Source: CAD feature listing. Evaluate the final solid. Frame: model axes, mm. A direction names the side the tool comes from. Round coordinates to 2 decimals unless told otherwise and drop trailing zeros. Loops run counter-clockwise (first coordinate to the right, second up) from the corner with the lowest first, then second, coordinate; pieces in that order, holes last. Notation, with made-up numbers: M 60.5,-33 L 101.5,-33 A22 cw 101.5,-17 Z; hole C -23,9 d10. An arc over 180 degrees is marked long. Answer as CSV lines item,"result". Start each with the question number.
```python
from build123d import *

# Parameters (mm, degrees)
SKETCH1_W           = 406.4
SKETCH1_H           = 431.8
SKETCH1_W_2         = 355.6
SKETCH1_H_2         = 381
BOSS_EXTRUDE1_DEPTH = 304.8
SKETCH2_W           = 254
SKETCH2_H           = 381
CUT_EXTRUDE1_DEPTH  = 552.975370827
BOSS_EXTRUDE2_DEPTH = 101.6
SKETCH4_W           = 25.4
SKETCH4_H           = 76.2
BOSS_EXTRUDE3_DEPTH = 533.4
BOSS_EXTRUDE4_DEPTH = 25.4
BOSS_EXTRUDE5_DEPTH = 25.4
SKETCH7_W           = 152.4
SKETCH7_H           = 25.4
BOSS_EXTRUDE6_DEPTH = 292.1
SKETCH8_R           = 4.7625
SKETCH8_R_2         = 7
CUT_EXTRUDE2_DEPTH  = 25.4
SKETCH9_R           = 12.7
CUT_EXTRUDE3_DEPTH  = 12.7
BOSS_EXTRUDE7_DEPTH = 25.4
SKETCH11_W          = 304.8
SKETCH11_H          = 25.4
BOSS_EXTRUDE8_DEPTH = 63.5
SKETCH12_W          = 304.8
SKETCH12_H          = 25.4
BOSS_EXTRUDE9_DEPTH = 63.5
SKETCH14_R          = 9.525
CUT_EXTRUDE4_DEPTH  = 830.495714275
SKETCH16_W          = 300
SKETCH16_H          = 160
CUT_EXTRUDE5_DEPTH  = 30


with BuildPart() as part:
    # Sketch1 → Boss-Extrude1 (new body)
    with BuildSketch(Plane.XY):
        Rectangle(SKETCH1_W, SKETCH1_H)
        Rectangle(SKETCH1_W_2, SKETCH1_H_2, mode=Mode.SUBTRACT)
    extrude(amount=BOSS_EXTRUDE1_DEPTH)

    # Sketch2 → Cut-Extrude1 (cut, through all)
    with BuildSketch(Plane(origin=(203.2, 0, 0), x_dir=(0, 0, -1), z_dir=(1, 0, 0))):
        with Locations((-177.8, 0)):
            Rectangle(SKETCH2_W, SKETCH2_H)
    extrude(amount=-CUT_EXTRUDE1_DEPTH, mode=Mode.SUBTRACT)

    # Sketch3 → Boss-Extrude2 (add)
    with BuildSketch(Plane(origin=(0, 215.9, 0), x_dir=(1, 0, 0), z_dir=(0, 1, 0))):
        Polygon((-57.785, 0), (-32.385, 0), (-32.385, -71.628), (32.385, -71.628), (32.385, 0), (57.785, 0), (57.785, -97.028), (32.385, -97.028), (-32.385, -97.028), (-57.785, -97.028), align=None)
    extrude(amount=BOSS_EXTRUDE2_DEPTH)

    # Sketch4 → Boss-Extrude3 (add)
    with BuildSketch(Plane.XZ.offset(215.9)):
        with Locations((-45.085, -38.1)):
            Rectangle(SKETCH4_W, SKETCH4_H)
        with Locations((45.085, -38.1)):
            Rectangle(SKETCH4_W, SKETCH4_H)
    extrude(amount=-BOSS_EXTRUDE3_DEPTH)

    # Sketch5 → Boss-Extrude4 (add)
    with BuildSketch(Plane.ZY.offset(57.785)):
        Polygon((-76.2, 317.5), (46.228, 508), (97.028, 508), (97.028, 317.5), align=None)
    extrude(amount=-BOSS_EXTRUDE4_DEPTH)

    # Sketch6 → Boss-Extrude5 (add)
    with BuildSketch(Plane(origin=(57.785, 0, 0), x_dir=(0, 0, -1), z_dir=(1, 0, 0))):
        Polygon((-46.228, 508), (-97.028, 508), (-97.028, 317.5), (76.2, 317.5), align=None)
    extrude(amount=-BOSS_EXTRUDE5_DEPTH)

    # Sketch7 → Boss-Extrude6 (add)
    with BuildSketch(Plane(origin=(0, 508, 0), x_dir=(1, 0, 0), z_dir=(0, 1, 0))):
        with Locations((0, -84.328)):
            Rectangle(SKETCH7_W, SKETCH7_H)
    extrude(amount=-BOSS_EXTRUDE6_DEPTH)

    # Sketch8 → Cut-Extrude2 (cut)
    with BuildSketch(Plane(origin=(0, 215.9, 0), x_dir=(1, 0, 0), z_dir=(0, 1, 0))):
        with Locations(Location((88.883, -229.362, 0), (0, 0, 270))):
            Circle(SKETCH8_R)
        with Locations(Location((57.5, -227.028, 0), (0, 0, 270))):
            Circle(SKETCH8_R_2)
        with Locations(Location((-88.917, -229.362, 0), (0, 0, 270))):
            Circle(SKETCH8_R)
        with Locations(Location((-57.5, -227.028, 0), (0, 0, 270))):
            Circle(SKETCH8_R_2)
        with Locations(Location((-88.917, -109.728, 0), (0, 0, 270))):
            Circle(SKETCH8_R)
        with Locations(Location((57.5, -112.028, 0), (0, 0, 270))):
            Circle(SKETCH8_R_2)
        with Locations(Location((88.883, -109.728, 0), (0, 0, 270))):
            Circle(SKETCH8_R)
        with Locations(Location((-57.5, -112.028, 0), (0, 0, 270))):
            Circle(SKETCH8_R_2)
    extrude(amount=-CUT_EXTRUDE2_DEPTH, mode=Mode.SUBTRACT)

    # Sketch9 → Cut-Extrude3 (cut)
    with BuildSketch(Plane.XZ.offset(-190.5)):
        with Locations(Location((-57.5, 227.028, 0), (0, 0, 270))):
            Circle(SKETCH9_R)
        with Locations(Location((57.5, 227.028, 0), (0, 0, 270))):
            Circle(SKETCH9_R)
        with Locations(Location((57.5, 112.028, 0), (0, 0, 270))):
            Circle(SKETCH9_R)
        with Locations(Location((-57.5, 112.028, 0), (0, 0, 270))):
            Circle(SKETCH9_R)
    extrude(amount=-CUT_EXTRUDE3_DEPTH, mode=Mode.SUBTRACT)

    # Sketch10 → Boss-Extrude7 (add)
    with BuildSketch(Plane(origin=(57.785, 0, 0), x_dir=(0, 0, -1), z_dir=(1, 0, 0))):
        Polygon((-71.628, 317.5), (76.2, 317.5), (-46.228, 508), (-71.628, 508), align=None)
    extrude(amount=-BOSS_EXTRUDE7_DEPTH)

    # Sketch11 → Boss-Extrude8 (add)
    with BuildSketch(Plane(origin=(203.2, 0, 0), x_dir=(0, 0, -1), z_dir=(1, 0, 0))):
        with Locations((-152.4, -203.2)):
            Rectangle(SKETCH11_W, SKETCH11_H)
    extrude(amount=BOSS_EXTRUDE8_DEPTH)

    # Sketch12 → Boss-Extrude9 (add)
    with BuildSketch(Plane.ZY.offset(203.2)):
        with Locations((152.4, -203.2)):
            Rectangle(SKETCH12_W, SKETCH12_H)
    extrude(amount=BOSS_EXTRUDE9_DEPTH)

    # Sketch14 → Cut-Extrude4 (cut, through all)
    with BuildSketch(Plane.XZ.offset(215.9)):
        with Locations(Location((-240.792, 213.978, 0), (0, 0, 270))):
            Circle(SKETCH14_R)
        with Locations(Location((-240.792, 125.078, 0), (0, 0, 90))):
            Circle(SKETCH14_R)
        with Locations(Location((240.792, 213.978, 0), (0, 0, 90))):
            Circle(SKETCH14_R)
        with Locations(Location((240.792, 125.078, 0), (0, 0, 270))):
            Circle(SKETCH14_R)
    extrude(amount=-CUT_EXTRUDE4_DEPTH, mode=Mode.SUBTRACT)

    # Sketch16 → Cut-Extrude5 (cut)
    with BuildSketch(Plane.XZ.offset(215.9)):
        with Locations((0, 174.8)):
            Rectangle(SKETCH16_W, SKETCH16_H)
    extrude(amount=-CUT_EXTRUDE5_DEPTH, mode=Mode.SUBTRACT)


solid = part.part
```
1) Section D-D, the plane z = 278.5. Return loops of the section in (x, y), and give its area (3 significant figures).
2) Contact query for flat-ended pins moving along their axis: pin 1 Ø8 at (x, y) = (-28.5, 4) entering from +Z; pin 2 Ø12 at (x, y) = (67, 35) entering from +Z; pin 3 Ø16 at (x, z) = (57.5, 227.028) entering from +Y; pin 4 Ø4 at (y, z) = (432.5, 5.5) entering from -X (3 decimals). Output: stop coordinate, or through.
3) Section C-C, the plane z = 159.5. Return loops of the section in (x, y), and give its area (3 significant figures).
4) Section A-A, the plane y = 133. Return loops of the section in (x, z) (3 decimals), and give its area (3 significant figures).
5) Mould query, pull axis X, two halves, no side actions, for faces 5 (the flat face through (-45.26, 411.42, -15.84)), 6 (the cylindrical face through (-56.942, 196.761, 124.716)). Classes: pulls with the +X half, pulls with the -X half, needs draft (parallel to the pull), parting line crosses it, or undercut.
6) Section B-B, the plane x = -120. Return loops of the section in (y, z), and give its area (3 significant figures).
7) Access query for faces 1 (the flat face through (-45, -3, 0)), 2 (the flat face through (-63, 203.2, 107)), 3 (the flat face through (-32.385, 151, -18)), 4 (the flat face through (45, 47, -76.2)). Directions: +Z, -Z, +X, -X, +Y, -Y. A direction counts if a zero-diameter tool reaches every point of the face in a straight line with its end or side. Return the directions, or none.
8) Ray query, line 1 along Z through (x, y) = (-57, 208); line 2 along Y through (x, z) = (46.5, 267.5); line 3 along X through (y, z) = (-142, -20) (3 decimals). Return the intervals inside material, ascending.
Findings below:
1,outline,"M -266.7,-215.9 L 266.7,-215.9 L 266.7,-190.5 L -266.7,-190.5 Z; M -203.2,190.5 L 203.2,190.5 L 203.2,215.9 L -203.2,215.9 Z"
1,area,"23,900 mm²"
2,pin 1,"z = 0"
2,pin 2,"through"
2,pin 3,"y = 215.9"
2,pin 4,"x = -57.785"
3,outline,"M -266.7,-215.9 L -150,-215.9 L -150,-190.5 L -266.7,-190.5 Z; M -203.2,190.5 L 203.2,190.5 L 203.2,215.9 L -203.2,215.9 Z; M 150,-215.9 L 266.7,-215.9 L 266.7,-190.5 L 150,-190.5 Z"
3,area,"16,300 mm²"
4,outline,"M -203.2,0 L -177.8,0 L -177.8,50.8 L -203.2,50.8 Z; M -57.785,-76.2 L -32.385,-76.2 L -32.385,0 L -57.785,0 Z; M 32.385,-76.2 L 57.785,-76.2 L 57.785,0 L 32.385,0 Z; M 177.8,0 L 203.2,0 L 203.2,50.8 L 177.8,50.8 Z"
4,area,"6,450 mm²"
5,face 5,"needs draft"
5,face 6,"undercut"
6,outline,"M -215.9,0 L -190.5,0 L -190.5,94.8 L -215.9,94.8 Z; M -215.9,254.8 L -190.5,254.8 L -190.5,304.8 L -215.9,304.8 Z; M 190.5,0 L 215.9,0 L 215.9,304.8 L 190.5,304.8 Z"
6,area,"11,400 mm²"
7,face 1,"+Z"
7,face 2,"-Y"
7,face 3,"-Z, +Y"
7,face 4,"-Z, +X, -X, +Y, -Y"
8,line 1,"-76.2 to 105.05, 119.01 to 220.05, 234.01 to 304.8"
8,line 2,"-215.9 to -190.5, 190.5 to 215.9"
8,line 3,"-57.785 to -32.385, 32.385 to 57.785"
